```python
from build123d import *

# Parameters (mm, degrees)
SKETCH1_R           = 6.8
BOSS_EXTRUDE1_DEPTH = 12.6
SKETCH2_R           = 5.8
CUT_EXTRUDE1_DEPTH  = 13.6
SKETCH3_R           = 12.4
BOSS_EXTRUDE3_DEPTH = 3
SKETCH4_R           = 2.35
CUT_EXTRUDE2_DEPTH  = 3
CUT_EXTRUDE3_DEPTH  = 3
CIRPATTERN1_COUNT   = 22
BOSS_EXTRUDE4_DEPTH = 10


with BuildPart() as part:
    # Sketch1 → Boss-Extrude1 (new body)
    with BuildSketch(Plane(origin=(0, 0, 0), x_dir=(1, 0, 0), z_dir=(0, 1, 0))):
        Circle(SKETCH1_R)
    extrude(amount=BOSS_EXTRUDE1_DEPTH)

    # Sketch2 → Cut-Extrude1 (cut, through all)
    with BuildSketch(Plane.XZ):
        Circle(SKETCH2_R)
    extrude(amount=-CUT_EXTRUDE1_DEPTH, mode=Mode.SUBTRACT)

    # Sketch3 → Boss-Extrude3 (add)
    with BuildSketch(Plane(origin=(0, 12.6, 0), x_dir=(1, 0, 0), z_dir=(0, 1, 0))):
        Circle(SKETCH3_R)
    extrude(amount=-BOSS_EXTRUDE3_DEPTH)

    # Sketch4 → Cut-Extrude2 (cut)
    with BuildSketch(Plane(origin=(0, 12.6, 0), x_dir=(1, 0, 0), z_dir=(0, 1, 0))):
        Circle(SKETCH4_R)
    extrude(amount=-CUT_EXTRUDE2_DEPTH, mode=Mode.SUBTRACT)

    # Sketch5 → Cut-Extrude3 (cut)
    with BuildSketch(Plane(origin=(0, 12.6, 0), x_dir=(1, 0, 0), z_dir=(0, 1, 0))):
        with BuildLine():
            ThreePointArc((12.308939841, -1.5), (12.4, 0), (12.308939841, 1.5))
            ThreePointArc((12.308939841, 1.5), (11.269957917, 0.865760233), (10.108939841, 0.5))
            ThreePointArc((10.108939841, 0.5), (9.773209975, 0), (10.108939841, -0.5))
            ThreePointArc((10.108939841, -0.5), (11.269957917, -0.865760233), (12.308939841, -1.5))
        make_face()
    cut_extrude3 = extrude(amount=-CUT_EXTRUDE3_DEPTH, mode=Mode.SUBTRACT)

    # CirPattern1: Cut-Extrude3 ×22 about axis
    cirpattern1_axis = Axis((0, 0, 0), (0, 1, 0))
    for i in range(1, CIRPATTERN1_COUNT):
        add(cut_extrude3.rotate(cirpattern1_axis, i * 360 / CIRPATTERN1_COUNT), mode=Mode.SUBTRACT)

    # Sketch6 → Boss-Extrude4 (add)
    with BuildSketch(Plane(origin=(0, 12.6, 0), x_dir=(1, 0, 0), z_dir=(0, 1, 0))):
        with BuildLine():
            Line((8.2, 0), (5.6, 0))
            ThreePointArc((5.6, 0), (5.105878964, -2.3), (3.710714286, -4.194114864))
            Line((3.710714286, -4.194114864), (5.433545918, -6.141382479))
            Line((5.433545918, -6.141382479), (6.332284818, -5.346229418))
            Line((6.332284818, -5.346229418), (5.333890775, -4.217773015))
            ThreePointArc((5.333890775, -4.217773015), (6.199995885, -2.792857143), (6.693280212, -1.2))
            Line((6.693280212, -1.2), (8.2, -1.2))
            Line((8.2, -1.2), (8.2, 0))
        make_face()
        with BuildLine():
            Line((-8.0353662, -1.634897558), (-7.796112899, -2.810804807))
            Line((-7.796112899, -2.810804807), (-6.319643965, -2.510398405))
            ThreePointArc((-6.319643965, -2.510398405), (-5.518683178, -3.972925369), (-4.385870591, -5.196550698))
            Line((-4.385870591, -5.196550698), (-5.139230485, -6.501408311))
            Line((-5.139230485, -6.501408311), (-4.1, -7.101408311))
            Line((-4.1, -7.101408311), (-2.8, -4.849742261))
            ThreePointArc((-2.8, -4.849742261), (-4.544797911, -3.271820892), (-5.487567161, -1.116515406))
            Line((-5.487567161, -1.116515406), (-8.0353662, -1.634897558))
        make_face()
        with BuildLine():
            Line((2.601820282, 7.776280037), (1.463828081, 8.157034225))
            Line((1.463828081, 8.157034225), (0.985753191, 6.728171419))
            ThreePointArc((0.985753191, 6.728171419), (-0.681312708, 6.765782512), (-2.307409622, 6.396550698))
            Line((-2.307409622, 6.396550698), (-3.060769515, 7.701408311))
            Line((-3.060769515, 7.701408311), (-4.1, 7.101408311))
            Line((-4.1, 7.101408311), (-2.8, 4.849742261))
            ThreePointArc((-2.8, 4.849742261), (-0.561081054, 5.571820892), (1.776852875, 5.310630269))
            Line((1.776852875, 5.310630269), (2.601820282, 7.776280037))
        make_face()
    extrude(amount=BOSS_EXTRUDE4_DEPTH)


solid = part.part
```
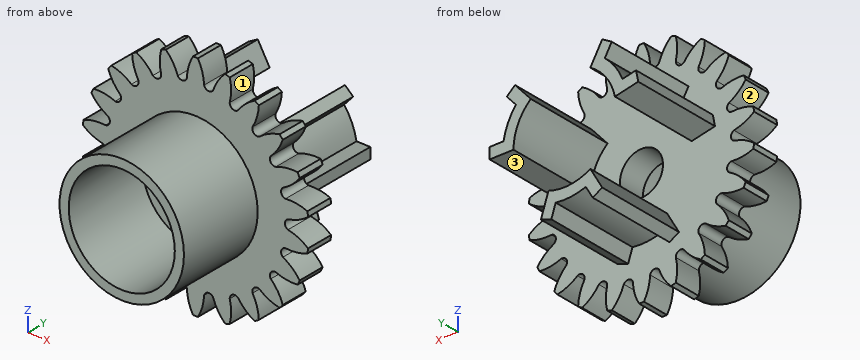
Model file for the job. Use its own axes, mm. Face numbers are marked on the shaded views. A direction names the side the tool comes from. Coordinates: 2 decimals unless noted, no trailing zeros. Order: outer loops, then holes, each group sorted by start corner. A loop starts at its lowest first (then second) coordinate and runs counter-clockwise, first axis right, second up. Notation, with made-up numbers: (-5.5, 1.25) -> (43.5, 1.25) arc R24 cw to (43.5, 18.25) -> close; hole circle Ø10 at (-6, -29.5). An arc over 180 degrees is marked (long way). Answer as a JSON object with one key per item and string values. Group by question number.
1) Drill centre lines: L1, parallel to X at y = 10.7, z = 0; L2, parallel to Z at x = 0, y = 10.45; L3, parallel to Z at x = 0, y = 5.25. Where is each one in solid material? Low to high.
2) Which spindle directions (+Z, -Z, +X, -X, +Y, -Y) get a long thin tool onto all of the face, cutting with end or side? Do the marked faces 1, 2 and 3. Say none if no direction does.
3) Cut at B-B, the plane x = 10.5. Write the cut outline in (y, z).
4) Flat gauge pins, fed straight in: pin 1 (4 mm diameter, centred on x = 7.5, y = 12, fed in from -Z); pin 2 (0.6 mm diameter, centred on y = 17.5, z = 0.5, fed in from +X); pin 3 (1.5 mm diameter, centred on x = 8, z = -7.5, fed in from -Y). Where does each tip first touch, or does it go through?
5) Cut at A-A, the plane y = 20.5. Write the cut outline in (x, z), then the cut area to 3 significant figures.
6) Cut at C-C, the plane y = 2. Write the cut outline in (x, z).
Check values:
{
 "1": {"L1": "x = -9.77 to -2.35, 2.35 to 9.77", "L2": "z = -12.4 to -2.35, 2.35 to 12.4", "L3": "z = -6.8 to -5.8, 5.8 to 6.8"},
 "2": {"face 1": "+Y, -Y", "face 2": "-X, +Y, -Y", "face 3": "-Z, +X, -X, +Y"},
 "3": {"outline": "(9.6, -5.41) -> (12.6, -5.41) -> (12.6, -3.95) -> (9.6, -3.95) -> close; (9.6, -2.39) -> (12.6, -2.39) -> (12.6, -0.59) -> (9.6, -0.59) -> close; (9.6, 0.59) -> (12.6, 0.59) -> (12.6, 2.39) -> (9.6, 2.39) -> close; (9.6, 3.95) -> (12.6, 3.95) -> (12.6, 5.41) -> (9.6, 5.41) -> close"},
 "4": {"pin 1": "stops at z = -10.57", "pin 2": "stops at x = 8.2", "pin 3": "stops at y = 9.6"},
 "5": {"outline": "(-8.04, 1.63) -> (-5.49, 1.12) arc R5.6 cw to (-2.8, 4.85) -> (-4.1, 7.1) -> (-5.14, 6.5) -> (-4.39, 5.2) arc R6.8 ccw to (-6.32, 2.51) -> (-7.8, 2.81) -> close; (-4.1, -7.1) -> (-3.06, -7.7) -> (-2.31, -6.4) arc R6.8 ccw to (0.99, -6.73) -> (1.46, -8.16) -> (2.6, -7.78) -> (1.78, -5.31) arc R5.6 cw to (-2.8, -4.85) -> close; (3.71, 4.19) arc R5.6 cw to (5.6, 0) -> (8.2, 0) -> (8.2, 1.2) -> (6.69, 1.2) arc R6.8 ccw to (5.33, 4.22) -> (6.33, 5.35) -> (5.43, 6.14) -> close", "area": "29.2 mm²"},
 "6": {"outline": "circle Ø13.6 at (0, 0); hole circle Ø11.6 at (0, 0)"}
}
